Design review of the part built by this model. Coordinates are the model's own, in mm. A direction names the side the tool comes from. Round coordinates to 2 decimals unless told otherwise and drop trailing zeros. Loops run counter-clockwise (first coordinate to the right, second up) from the corner with the lowest first, then second, coordinate; pieces in that order, holes last. Notation, with made-up numbers: (-17, 45) - (-12, 45) arc R25 ccw to (-12, 64) - close; hole circle Ø7 at (-7.75, 23). An arc over 180 degrees is marked (long way). Use one line per item in the form item = value. Start each with the question number.
(1) The part is to be moulded in two halves that separate along Y. For faces 4 (the cylindrical face through (-0.065, -3.174, 9.409)), 5 (the flat face through (0, -5, 0)), say which applies: released by +Y, released by -Y, zero draft, split by the parting line, or undercut.
(2) Wall thickness on probe 1 along Y at (x, z) = (0.25, 10.25); probe 2 along X at (y, z) = (-2, 17.5); probe 3 along Y at (x, z) = (3.5, 9.75): over which ranges is each line inside the solid? List them lowest first. Write a range as [from, to].
(3) We need section A-A, the plane x = 0. Write out the cut boundary in (y, z) (3 decimals).
(4) Machinability: for faces 1 (the cylindrical face through (0.065, 3.174, 9.409)), 2 (the flat face through (0, -5, 19.05)), 3 (the flat face through (-7, -0.318, 10)), which of the approach directions +Z, -Z, +X, -X, +Y, -Y give a long, thin tool a straight path to every point of the face, cutting with its end or side? Answer none if there is none.
(5) We need section C-C, the plane x = -6.25. Write out the cut boundary in (y, z).
(6) We need section D-D, the plane y = -5. Write out the cut boundary in (x, z).
(7) For pin 1 (10 mm diameter, centred on x = 6.5, y = -7, fed in from -Z); pin 2 (0.5 mm diameter, centred on y = 0, z = 14, fed in from -X); pin 3 (3 mm diameter, centred on y = 2.5, z = 11, fed in from -X); pin 4 (3 mm diameter, centred on y = -2, z = 10, fed in from +X), all flat-tipped, find the tip position at first contact; note any pin that passes through.
from build123d import *

# Parameters (mm, degrees)
SKETCH1_R           = 11.049
SKETCH1_R_2         = 3.175
BOSS_EXTRUDE1_DEPTH = 19.05
FILLET1_R           = 1.27
SKETCH3_W           = 21.529859436
SKETCH3_H           = 0.635
CUT_EXTRUDE1_DEPTH  = 20.05


with BuildPart() as part:
    # Sketch1 → Boss-Extrude1 (new body)
    with BuildSketch(Plane.XY):
        Circle(SKETCH1_R)
        Circle(SKETCH1_R_2, mode=Mode.SUBTRACT)
    extrude(amount=BOSS_EXTRUDE1_DEPTH)

    # Fillet1
    fillet1_edges = [part.edges().sort_by_distance(p)[0] for p in [
        (-3.175, 0, 0),
        (-3.175, 0, 19.05),
    ]]
    fillet(fillet1_edges, radius=FILLET1_R)

    # Sketch3 → Cut-Extrude1 (cut, through all)
    with BuildSketch(Plane.XY.offset(19.05)):
        with Locations((-0.784069021, 0)):
            Rectangle(SKETCH3_W, SKETCH3_H)
    extrude(amount=-CUT_EXTRUDE1_DEPTH, mode=Mode.SUBTRACT)


solid = part.part
Data:
q1.face_4 = undercut
q1.face_5 = zero draft
q2.probe_1 = [-11.05, -3.17], [3.17, 11.05]
q2.probe_2 = [-10.87, -2.47], [2.47, 10.87]
q2.probe_3 = [-10.48, -0.32], [0.32, 10.48]
q3.outline = (-11.049, 0) - (-4.445, 0) arc R1.27 ccw to (-3.175, 1.27) - (-3.175, 17.78) arc R1.27 ccw to (-4.445, 19.05) - (-11.049, 19.05) - close; (3.175, 1.27) arc R1.27 ccw to (4.445, 0) - (11.049, 0) - (11.049, 19.05) - (4.445, 19.05) arc R1.27 ccw to (3.175, 17.78) - close
q4.face_1 = +Z, -Z
q4.face_2 = +Z, +X, -X, +Y, -Y
q4.face_3 = +Z, -Z, -X
q5.outline = (-9.11, 0) - (-0.32, 0) - (-0.32, 19.05) - (-9.11, 19.05) - close; (0.32, 0) - (9.11, 0) - (9.11, 19.05) - (0.32, 19.05) - close
q6.outline = (-9.85, 0) - (9.85, 0) - (9.85, 19.05) - (-9.85, 19.05) - close
q7.pin_1 = 0
q7.pin_2 = 9.98
q7.pin_3 = -11
q7.pin_4 = 11.04
